Build history of the part. All positions in model axes, mm. A direction names the side the tool comes from. Give positions to 0.01 mm unless a question says otherwise; leave off trailing zeros. Write each loop counter-clockwise with the first axis right and the second up, starting at its lowest first coordinate (ties: lowest second). Pieces come first, ordered by that corner, then holes. Notation, with made-up numbers: M -8.75,66.5 L 20.25,66.5 A17 ccw 20.25,88.5 Z; hole C 47.5,38.25 d11. An arc over 180 degrees is marked long. One line per item, written item: value. Start each with the question number.
from build123d import *

# Parameters (mm, degrees)
F0_W          = 10
F0_H          = 10
F0_W_2        = 9
F0_H_2        = 9
F1_DEPTH      = 37.5
F1_DEPTH_BACK = 37.5
F2_R          = 2.5
F3_DEPTH      = 10
F4_R          = 2.5
F5_DEPTH      = 10


with BuildPart() as f1:
    # F0 (on Right) → F1 (new body, two sides)
    with BuildSketch(Plane.YZ) as f1_sk:
        Rectangle(F0_W, F0_H)
        Rectangle(F0_W_2, F0_H_2, mode=Mode.SUBTRACT)
    extrude(amount=F1_DEPTH)
    extrude(f1_sk.sketch, amount=-F1_DEPTH_BACK)

    # F2 (on face) → F3 (cut)
    with BuildSketch(Plane.XY.offset(5)):
        with Locations((-24, 0)):
            Circle(F2_R)
        with Locations((24, 0)):
            Circle(F2_R)
    extrude(amount=-F3_DEPTH, mode=Mode.SUBTRACT)

    # F4 (on face) → F5 (cut)
    with BuildSketch(Plane.XZ.offset(5)):
        with Locations((-28, 0)):
            Circle(F4_R)
        with Locations((28, 0)):
            Circle(F4_R)
    extrude(amount=-F5_DEPTH, mode=Mode.SUBTRACT)


solid = f1.part
1) Band-saw the part on B-B (z = 3.75). List the corners of the cut face in (x, y), then the cut area to 3 significant figures.
2) Tool access for faces 1 (the face through (25.5, -4.8, 0.1)), 2 (the face through (1, 0, 4.5)): list every direction of +Z, -Z, +X, -X, +Y, -Y with a clear straight run to the whole face (end or side of a thin tool).
3) Band-saw the part on D-D (x = -11.5). List the corners of the cut face in (y, z), then the cut area to 3 significant figures.
4) Mould opens along X. For faces 3 (the face through (-26.5, 0.1, -4.7)), 4 (the face through (1, 0, -4.5)), 5 (the face through (37.5, -0.4, -4.8)) say: released by +X, released by -X, zero draft, split by the parting line, or undercut.
5) Drop a flat-ended pin along its axis: P1, Ø4.5, axis at x = -24, y = 0, coming from the -Z side. Give the stop position or say it passes through.
6) Band-saw the part on A-A (x = -28). List the corners of the cut face in (y, z).
7) Probe line 1 along Z through (x, y) = (-28, -4.75); line 2 along Y through (x, z) = (13, 0.5). List the from-to ranges inside material, lowest first. Write a range as from..to.
Model answer:
1. outline: M -37.5,-5 L 37.5,-5 L 37.5,-4.5 L -37.5,-4.5 Z; M -37.5,4.5 L 37.5,4.5 L 37.5,5 L -37.5,5 Z
1. area: 75.0 mm²
2. face 1: +Y, -Y
2. face 2: +X, -X
3. outline: M -5,-5 L 5,-5 L 5,5 L -5,5 Z; hole M -4.5,-4.5 L 4.5,-4.5 L 4.5,4.5 L -4.5,4.5 Z
3. area: 19.0 mm²
4. face 3: undercut
4. face 4: zero draft
4. face 5: released by +X
5. P1: passes through
6. outline: M -5,-5 L 5,-5 L 5,-2.5 L 4.5,-2.5 L 4.5,-4.5 L -4.5,-4.5 L -4.5,-2.5 L -5,-2.5 Z; M -5,2.5 L -4.5,2.5 L -4.5,4.5 L 4.5,4.5 L 4.5,2.5 L 5,2.5 L 5,5 L -5,5 Z
7. line 1: z = -5..-2.5, 2.5..5
7. line 2: y = -5..-4.5, 4.5..5
